from build123d import *

# Parameters (mm, degrees)
CROQUIS1_W              = 165
CROQUIS1_H              = 20
SALIENTE_EXTRUIR1_DEPTH = 178
CORTAR_EXTRUIR1_REACH   = 401.805
CROQUIS2_R              = 20.190307202


with BuildPart() as part:
    # Croquis1 → Saliente-Extruir1 (new body)
    with BuildSketch(Plane(origin=(0, 0, 360), x_dir=(-1, 0, 0), z_dir=(0, 0, -1))):
        with Locations((-74.745907017, -157.165586138)):
            Rectangle(CROQUIS1_W, CROQUIS1_H)
        with Locations((90.254092983, -157.165586138)):
            Rectangle(CROQUIS1_W, CROQUIS1_H)
    extrude(amount=SALIENTE_EXTRUIR1_DEPTH)

    # Croquis2 → Cortar-Extruir1 (cut, up to next)
    with BuildSketch(Plane.XZ.offset(167.165586138), mode=Mode.PRIVATE) as cortar_extruir1_sk1:
        with Locations((-104.519454625, 319.809692798)):
            Circle(CROQUIS2_R)
    cortar_extruir1_tool1 = extrude(cortar_extruir1_sk1.sketch, amount=-CORTAR_EXTRUIR1_REACH, mode=Mode.PRIVATE) & part.part
    # Croquis2 → Cortar-Extruir1 (cut, up to next)
    with BuildSketch(Plane.XZ.offset(167.165586138), mode=Mode.PRIVATE) as cortar_extruir1_sk2:
        with Locations((-7.754092983, 319.809692798)):
            Circle(CROQUIS2_R)
    cortar_extruir1_tool2 = extrude(cortar_extruir1_sk2.sketch, amount=-CORTAR_EXTRUIR1_REACH, mode=Mode.PRIVATE) & part.part
    # Croquis2 → Cortar-Extruir1 (cut, up to next)
    with BuildSketch(Plane.XZ.offset(167.165586138), mode=Mode.PRIVATE) as cortar_extruir1_sk3:
        with Locations((89.011268658, 319.809692798)):
            Circle(CROQUIS2_R)
    cortar_extruir1_tool3 = extrude(cortar_extruir1_sk3.sketch, amount=-CORTAR_EXTRUIR1_REACH, mode=Mode.PRIVATE) & part.part
    add(cortar_extruir1_tool1.solids().sort_by_distance((-104.519455, -167.165586, 319.809693))[0], mode=Mode.SUBTRACT)
    add(cortar_extruir1_tool2.solids().sort_by_distance((-7.754093, -167.165586, 319.809693))[0], mode=Mode.SUBTRACT)
    add(cortar_extruir1_tool3.solids().sort_by_distance((89.011269, -167.165586, 319.809693))[0], mode=Mode.SUBTRACT)


solid = part.part
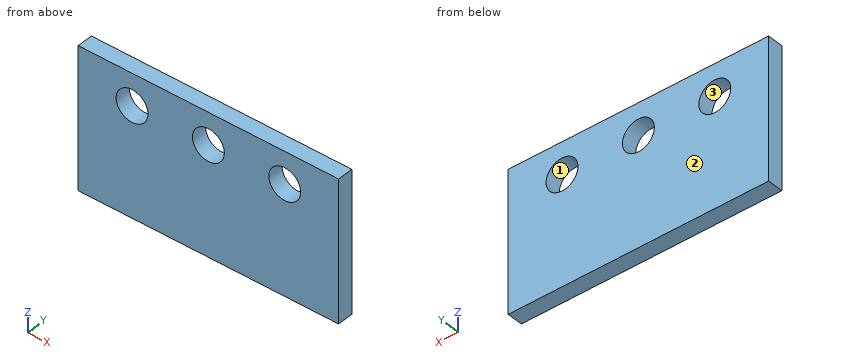
Part model, mm, in its own coordinate system. Face numbers are marked on the shaded views. Coordinates: 2 decimals unless noted, no trailing zeros. Write each loop counter-clockwise with the first axis right and the second up, starting at its lowest first coordinate (ties: lowest second). Pieces come first, ordered by that corner, then holes. Notation, with made-up numbers: M 27.5,10 L 49.5,10 A24 ccw 49.5,46 Z; hole C 75.5,31.25 d7. An arc over 180 degrees is marked long. Return JSON: item names as keys, results as strings.
1. Probe L1, parallel to X at y = -158, z = 320.5; L2, parallel to X at y = -150.5, z = 326; L3, parallel to Z at x = 95, y = -165.5. List the from-to ranges inside material, lowest first.
Determined:
{"L1": "-172.75 to -124.7, -84.34 to -27.93, 12.42 to 68.83, 109.19 to 157.25", "L2": "-172.75 to -123.74, -85.3 to -26.97, 11.46 to 69.79, 108.23 to 157.25", "L3": "182 to 300.53, 339.09 to 360"}
2. Saw through at C-C, the plane y = -158.5. Write the cut outline in (x, z).
Determined:
{"outline": "M -172.75,182 L 157.25,182 L 157.25,360 L -172.75,360 Z; hole C -104.52,319.81 d40.38; hole C -7.75,319.81 d40.38; hole C 89.01,319.81 d40.38"}
3. Flat gauge pin, fed straight in: pin 1 Ø24 at (x, z) = (-7.75, 319.81) entering from -Y. Where does the tip first touch, or does it go through?
Determined:
{"pin 1": "through"}
4. Saw through at A-A, the plane z = 325. Write the cut outline in (x, y), then the cut area to 3 significant figures.
Determined:
{"outline": "M -172.75,-167.17 L -124.03,-167.17 L -124.03,-147.17 L -172.75,-147.17 Z; M -85.01,-167.17 L -27.27,-167.17 L -27.27,-147.17 L -85.01,-147.17 Z; M 11.76,-167.17 L 69.5,-167.17 L 69.5,-147.17 L 11.76,-147.17 Z; M 108.52,-167.17 L 157.25,-167.17 L 157.25,-147.17 L 108.52,-147.17 Z", "area": "4,260 mm²"}
5. Saw through at B-B, the plane x = -20. Write the cut outline in (y, z).
Determined:
{"outline": "M -167.17,182 L -147.17,182 L -147.17,303.76 L -167.17,303.76 Z; M -167.17,335.86 L -147.17,335.86 L -147.17,360 L -167.17,360 Z"}
6. Pull direction Z, two halves, no side cores. Call the marked faces 1, 2 and 3: pulls with the +Z half, pulls with the -Z half, needs draft (parallel to the pull), parting line crosses it, or undercut.
Determined:
{"face 1": "undercut", "face 2": "needs draft", "face 3": "undercut"}
